```python
from build123d import *

# Parameters (mm, degrees)
F0_W     = 104.999994
F0_H     = 59.99988
F1_DEPTH = 20.000011
F2_R     = 7.5
F2_R_2   = 7.507622
F3_DEPTH = 20.001011
F4_R     = 2.5


with BuildPart() as f1:
    # F0 (on Top) → F1 (new body)
    with BuildSketch(Plane.XY):
        Rectangle(F0_W, F0_H)
    extrude(amount=F1_DEPTH)

    # F2 (on Top) → F3 (cut, through all)
    with BuildSketch(Plane.XY):
        Circle(F2_R)
        with Locations((-25, 0)):
            Circle(F2_R_2)
        with Locations((25, 0)):
            Circle(F2_R_2)
    extrude(amount=F3_DEPTH, mode=Mode.SUBTRACT)

    # F4
    f4_edges = [f1.edges().sort_by_distance(p)[0] for p in [
        (0, 29.99994, 0),
        (52.499997, 0, 0),
        (0, -29.99994, 0),
        (-52.499997, 0, 0),
        (0, 29.99994, 20.000011),
        (52.499997, 0, 20.000011),
        (0, -29.99994, 20.000011),
        (-52.499997, 0, 20.000011),
    ]]
    fillet(f4_edges, radius=F4_R)


solid = f1.part
```
Read the model definition and answer for the solid it produces. Units are mm, in the model's axes. Give positions to 0.01 mm unless a question says otherwise; leave off trailing zeros. Write each loop counter-clockwise with the first axis right and the second up, starting at its lowest first coordinate (ties: lowest second). Pieces come first, ordered by that corner, then holes. Notation, with made-up numbers: (-13.75, 35.5) - (18.25, 35.5) arc R18 cw to (18.25, 46.5) - close; hole circle Ø10 at (17, 28). An arc over 180 degrees is marked (long way). Write item = value, one per line. Start each with the question number.
Item 1: Find section A-A (x = 0). Give the vertices of the cut face in (y, z), then the cut area to 3 significant figures.
Item 2: This flat-tipped pin is pushed along its axis until it touches: P1, Ø19.5, axis at x = 0, y = 0, coming from the +Z side. Where does it stop, or does it pass through?
Item 3: Find the intervals of material crossed by probe 1 along X at (y, z) = (0, 15); probe 2 along Y at (x, z) = (0, 6.5); probe 3 along X at (y, z) = (-4.5, 8.25), in increasing order. Write a range as [from, to].
Item 4: Find section D-D (x = 25). Give the vertices of the cut face in (y, z), then the cut area to 3 significant figures.
Item 5: Find section C-C (z = 12.25). Give the vertices of the cut face in (x, y), then the cut area to 3 significant figures.
Item 6: Find section B-B (y = 0). Give the vertices of the cut face in (x, z), then the cut area to 3 significant figures.
Item 7: The mould has two halves that part along Y. Classify faces 1 (the cylindrical face through (-7.493, 0.33, 9.86)), 2 (the cylindrical face through (-30.958, -4.568, 9.86)), 3 (the cylindrical face through (0.735, -29.287, 0.752)), 4 (the flat face through (52.5, 0, 10)): +Y half, -Y half, draft (parallel to the pull), parting line (faces both ways), or undercut.
Response:
q1.outline = (-30, 2.5) arc R2.5 ccw to (-27.5, 0) - (-7.5, 0) - (-7.5, 20) - (-27.5, 20) arc R2.5 ccw to (-30, 17.5) - close; (7.5, 0) - (27.5, 0) arc R2.5 ccw to (30, 2.5) - (30, 17.5) arc R2.5 ccw to (27.5, 20) - (7.5, 20) - close
q1.area = 895 mm²
q2.P1 = 20
q3.probe_1 = [-52.5, -32.51], [-17.49, -7.5], [7.5, 17.49], [32.51, 52.5]
q3.probe_2 = [-30, -7.5], [7.5, 30]
q3.probe_3 = [-52.5, -31.01], [-18.99, -6], [6, 18.99], [31.01, 52.5]
q4.outline = (-30, 2.5) arc R2.5 ccw to (-27.5, 0) - (-7.51, 0) - (-7.51, 20) - (-27.5, 20) arc R2.5 ccw to (-30, 17.5) - close; (7.51, 0) - (27.5, 0) arc R2.5 ccw to (30, 2.5) - (30, 17.5) arc R2.5 ccw to (27.5, 20) - (7.51, 20) - close
q4.area = 894 mm²
q5.outline = (-52.5, -30) - (52.5, -30) - (52.5, 30) - (-52.5, 30) - close; hole circle Ø15.02 at (-25, 0); hole circle Ø15 at (0, 0); hole circle Ø15.02 at (25, 0)
q5.area = 5,770 mm²
q6.outline = (-52.5, 2.5) arc R2.5 ccw to (-50, 0) - (-32.51, 0) - (-32.51, 20) - (-50, 20) arc R2.5 ccw to (-52.5, 17.5) - close; (-17.49, 0) - (-7.5, 0) - (-7.5, 20) - (-17.49, 20) - close; (7.5, 0) - (17.49, 0) - (17.49, 20) - (7.5, 20) - close; (32.51, 0) - (50, 0) arc R2.5 ccw to (52.5, 2.5) - (52.5, 17.5) arc R2.5 ccw to (50, 20) - (32.51, 20) - close
q6.area = 1,190 mm²
q7.face_1 = undercut
q7.face_2 = undercut
q7.face_3 = -Y half
q7.face_4 = draft
